Drawing for the job (mm, zero at the part's lowest x, y, z). A direction names the side the tool comes from. Give positions to 0.01 mm unless a question says otherwise; leave off trailing zeros. Write each loop counter-clockwise with the first axis right and the second up, starting at its lowest first coordinate (ties: lowest second). Pieces come first, ordered by that corner, then holes. Notation, with made-up numbers: (1, 42.25) - (34, 42.25) arc R22 ccw to (34, 57.25) - close; hole circle Ø2 at (39, -4). An arc over 180 degrees is marked (long way). Use CSV: the item, a comma, the result in double quotes.
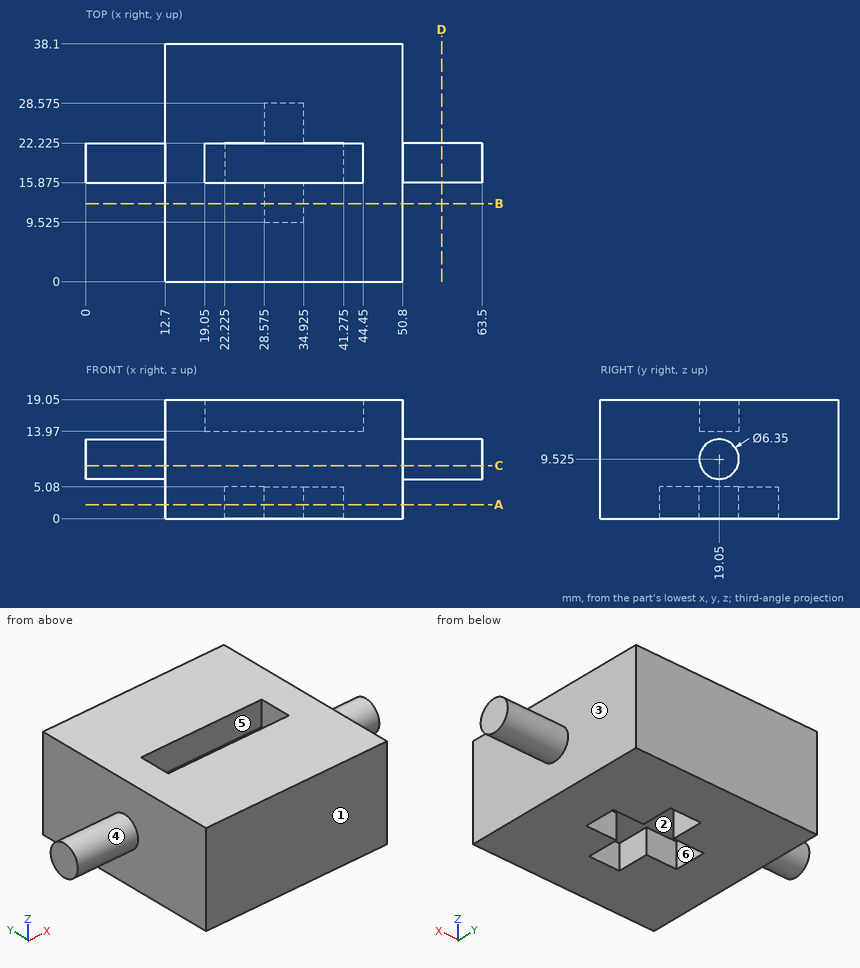
(1) Saw through at C-C, the plane z = 8.5. List the corners of the cut face in (x, y) (3 decimals).
Checked values:
outline,"(0, 16.045) - (12.7, 16.045) - (12.7, 0) - (50.8, 0) - (50.8, 16.045) - (63.5, 16.045) - (63.5, 22.055) - (50.8, 22.055) - (50.8, 38.1) - (12.7, 38.1) - (12.7, 22.055) - (0, 22.055) - close"
(2) Flat gauge pins, fed straight in: P1, Ø5, axis at x = 34, y = 19.5, coming from the +Z side; P2, Ø2.5, axis at y = 25.5, z = 2, coming from the -X side; P3, Ø6, axis at y = 34, z = 15.5, coming from the +X side. Where does each tip first touch, or does it go through?
Checked values:
P1,"stops at z = 13.97"
P2,"stops at x = 12.7"
P3,"stops at x = 50.8"
(3) 3-axis set-ups, long thin cutter, end or side, ignore diameter. For the marked faces 4, 5 and 6: which of +Z, -Z, +X, -X, +Y, -Y reach the whole face in a straight line?
Checked values:
face 4,"-X"
face 5,"+Z"
face 6,"-Z"
(4) Wall check: probe 1 along X at (y, z) = (11, 2.5) (3 decimals); probe 2 along Z at (x, y) = (32, 12); probe 3 along X at (y, z) = (7, 18). Give the ranges that are in metal, low to high. Write a range as [from, to].
Checked values:
probe 1,"x = [12.7, 28.575], [34.925, 50.8]"
probe 2,"z = [5.08, 19.05]"
probe 3,"x = [12.7, 50.8]"
(5) Saw through at A-A, the plane z = 2.25. List the corners of the cut face in (x, y) (3 decimals).
Checked values:
outline,"(12.7, 0) - (50.8, 0) - (50.8, 38.1) - (12.7, 38.1) - close; hole (22.225, 15.875) - (28.575, 15.875) - (28.575, 9.525) - (34.925, 9.525) - (34.925, 15.875) - (41.275, 15.875) - (41.275, 22.225) - (34.925, 22.225) - (34.925, 28.575) - (28.575, 28.575) - (28.575, 22.225) - (22.225, 22.225) - close"
(6) Saw through at D-D, the plane x = 57. List the corners of the cut face in (y, z) (3 decimals).
Checked values:
outline,"circle Ø6.35 at (19.05, 9.525)"
(7) Saw through at B-B, the plane y = 12.5. List the corners of the cut face in (x, z) (3 decimals), then the cut area to 3 significant figures.
Checked values:
outline,"(12.7, 0) - (28.575, 0) - (28.575, 5.08) - (34.925, 5.08) - (34.925, 0) - (50.8, 0) - (50.8, 19.05) - (12.7, 19.05) - close"
area,"694 mm^2"
(8) Pull direction X, two halves, no side cores. Call the marked faces 1, 2 and 3: released by +X, released by -X, zero draft, split by the parting line, or undercut.
Checked values:
face 1,"zero draft"
face 2,"undercut"
face 3,"released by +X"
